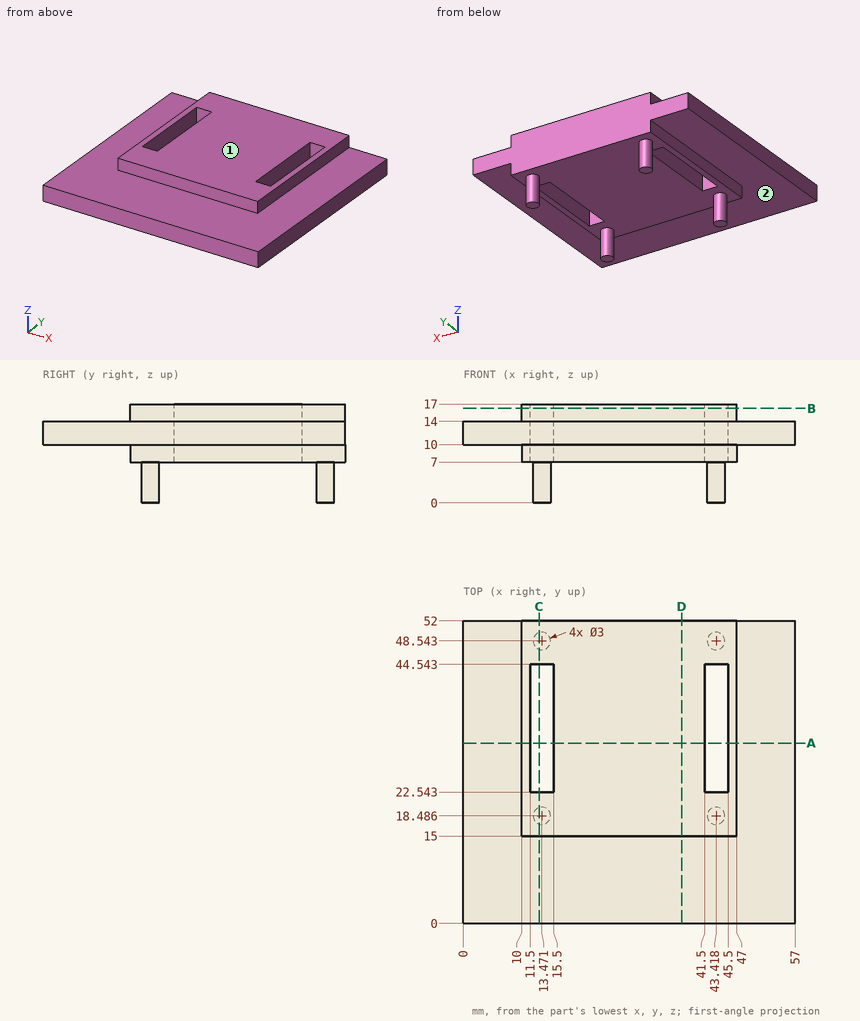
Drawing for the job (mm, zero at the part's lowest x, y, z). A direction names the side the tool comes from. Round coordinates to 2 decimals unless told otherwise and drop trailing zeros. Loops run counter-clockwise (first coordinate to the right, second up) from the corner with the lowest first, then second, coordinate; pieces in that order, holes last.
1. Band-saw the part on D-D, the plane x = 37.5. List the corners of the cut face in (y, z), and give its area (3 significant figures).
Check values:
outline: (0, 10) - (15, 10) - (15, 7) - (52, 7) - (52, 17) - (15, 17) - (15, 14) - (0, 14) - close
area: 430 mm2
2. Wall check: probe 1 along X at (y, z) = (36.5, 10.5); probe 2 along X at (y, z) = (30, 8.75); probe 3 along Y at (x, z) = (45, 12.75). Give the ranges that are in metal, low to high.
Check values:
probe 1: x = 0 to 11.5, 15.5 to 41.5, 45.5 to 57
probe 2: x = 10 to 11.5, 15.5 to 41.5, 45.5 to 47
probe 3: y = 0 to 22.54, 44.54 to 52
3. Band-saw the part on C-C, the plane x = 13. List the corners of the cut face in (y, z), and give its area (3 significant figures).
Check values:
outline: (0, 10) - (15, 10) - (15, 7) - (17.06, 7) - (17.06, 0) - (19.91, 0) - (19.91, 7) - (22.54, 7) - (22.54, 17) - (15, 17) - (15, 14) - (0, 14) - close; (44.54, 7) - (47.12, 7) - (47.12, 0) - (49.97, 0) - (49.97, 7) - (52, 7) - (52, 17) - (44.54, 17) - close
area: 250 mm2
4. Drop flat-ended pins along their axis: P1, Ø2.5, axis at y = 40.5, z = 15, coming from the +X side; P2, Ø2.5, axis at y = 38.5, z = 8.5, coming from the -X side; P3, Ø1.5, axis at y = 24.5, z = 9, coming from the +X side; P4, Ø3, axis at x = 15, y = 44.5, coming from the -Z side. Give the stop position or say it passes through.
Check values:
P1: stops at x = 57
P2: stops at x = 10
P3: stops at x = 47
P4: stops at z = 7
5. Band-saw the part on B-B, the plane z = 16.25. List the corners of the cut face in (x, y), and give its area (3 significant figures).
Check values:
outline: (10, 15) - (47, 15) - (47, 52) - (10, 52) - close; hole (11.5, 22.54) - (15.5, 22.54) - (15.5, 44.54) - (11.5, 44.54) - close; hole (41.5, 22.54) - (45.5, 22.54) - (45.5, 44.54) - (41.5, 44.54) - close
area: 1,190 mm2
6. Band-saw the part on A-A, the plane y = 31. List the corners of the cut face in (x, z).
Check values:
outline: (0, 10) - (10, 10) - (10, 7) - (11.5, 7) - (11.5, 17) - (10, 17) - (10, 14) - (0, 14) - close; (15.5, 7) - (41.5, 7) - (41.5, 17) - (15.5, 17) - close; (45.5, 7) - (47, 7) - (47, 10) - (57, 10) - (57, 14) - (47, 14) - (47, 17) - (45.5, 17) - close
7. Tool access for the marked faces 1 and 2: list every direction of +Z, -Z, +X, -X, +Y, -Y with a clear straight run to the whole face (end or side of a thin tool).
Check values:
face 1: +Z, +X, -X, +Y, -Y
face 2: -Z, -Y
